Autodesk Inventor part; units mm, degrees
ref_plane "Work Plane4" through (-230, -208.6603, 455) normal (0, 0.8660254, -0.5) x (1, 0, 0)
ref_plane "Work Plane5" through (-230, -200, 450) normal (0, 0.7660444, -0.6427876) x (1, 0, 0)
ref_plane "YZ Plane" through (0, 0, 0) normal (1, 0, 0) x (0, 1, 0)
sketch "Sketch1" plane through (0, 0, 0) normal (0, 0, 1) x (1, 0, 0)
  line L0 (230, -200) -> (-230, -200)
  line L1 (-230, -200) -> (-230, 200)
  line L2 (-230, 200) -> (230, 200)
  line L3 (230, 200) -> (230, -200)
  line L4 (230, -200) -> (-230, 200) construction
  line L5 (-230, -200) -> (230, 200) construction
  line L6 (-190, 200) -> (-160.6372, 250.8579)
  line L7 (-160.6372, 250.8579) -> (139.1421, 250.8579)
  line L8 (139.1421, 250.8579) -> (190, 200)
  line L9 (139.1421, 250.8579) -> (122.8634, 211.5574) construction
  line L10 (135, 250.8579) -> (135, 240.8579) construction
  line L11 (230, 200) -> (190, 200)
  line L12 (190, 200) -> (190, 160)
  line L13 (190, 160) -> (230, 160)
  line L14 (230, 160) -> (230, 200)
  line L15 (-150, 110) -> (150, 110)
  line L16 (150, 110) -> (150, -140)
  line L17 (150, -140) -> (-150, -140)
  line L18 (-150, -140) -> (-150, 110)
  line L19 (-230, -200) -> (-190, -200)
  line L20 (-190, -200) -> (-190, -160)
  line L21 (-190, -160) -> (-230, -160)
  line L22 (-230, -160) -> (-230, -200)
  line L23 (230, -200) -> (190, -200)
  line L24 (190, -200) -> (190, -160)
  line L25 (190, -160) -> (230, -160)
  line L26 (230, -160) -> (230, -200)
  line L27 (-230, 200) -> (-190, 200)
  line L28 (-190, 200) -> (-190, 160)
  line L29 (-190, 160) -> (-230, 160)
  line L30 (-230, 160) -> (-230, 200)
  line L31 (-40, 200) -> (40, 200)
  line L32 (40, 200) -> (40, 160)
  line L33 (40, 160) -> (-40, 160)
  line L34 (-40, 160) -> (-40, 200)
  line L35 (125, 250.8579) -> (135, 250.8579)
  line L36 (135, 250.8579) -> (135, 230.8579)
  line L37 (135, 230.8579) -> (125, 230.8579)
  line L38 (125, 230.8579) -> (125, 250.8579)
  line L39 (149.1421, 240.8579) -> (142.0711, 247.9289)
  line L40 (142.0711, 247.9289) -> (127.9289, 233.7868)
  line L41 (127.9289, 233.7868) -> (134.2929, 227.4228)
  line L42 (135.7071, 227.4228) -> (149.1421, 240.8579)
  line L43 (135, 200) -> (132, 200)
  line L44 (132, 200) -> (132, 239)
  line L45 (132, 239) -> (135, 239)
  line L46 (135, 239) -> (135, 200)
  line L47 (135, 200) -> (95, 200)
  line L48 (95, 200) -> (95, 180)
  line L49 (95, 180) -> (135, 180)
  line L50 (135, 180) -> (135, 200)
  line L51 (-222, 80) -> (-132, 80)
  line L52 (-132, 80) -> (-132, -140)
  line L53 (-132, -140) -> (-222, -140)
  line L54 (-222, -140) -> (-222, 80)
  circle A0 centre (-112, -40) radius 100
  circle A1 centre (112, -40) radius 100
  line L55 (-230, -40) -> (230, -40) construction
  line L56 (-112, -40) -> (112, -40)
  arc A2 (134.2929, 227.4228) -> (135.7071, 227.4228) centre (135, 228.1299) ccw
  point P0 (0, 0)
  point P1 (0, 110)
  point P2 (0, 200)
  point P3 (135, 226.7157)
  point P4 (0, -40)
  dimension "d0" = 460
  dimension "d1" = 400
  dimension "d2" = 40
  dimension "d3" = 40
  dimension "d4" = 120
  dimension "d5" = 135
  dimension "d30" = 67.5
  dimension "d32" = 10
  dimension "d34" = 50.8579
  dimension "d35" = 40
  dimension "d36" = 40
  dimension "d37" = 300
  dimension "d38" = 250
  dimension "d39" = 60
  dimension "d40" = 40
  dimension "d41" = 40
  dimension "d42" = 40
  dimension "d43" = 40
  dimension "d44" = 40
  dimension "d45" = 40
  dimension "d46" = 80
  dimension "d47" = 40
  dimension "d48" = 10
  dimension "d50" = 10
  dimension "d51" = 3
  dimension "d52" = 39
  dimension "d53" = 40
  dimension "d54" = 20
  dimension "d55" = 55
  dimension "d56" = 105
  dimension "d57" = 90
  dimension "d58" = 220
  dimension "d59" = 8
  dimension "d60" = 20
  dimension "d61" = 55
  dimension "d63" = 200
  dimension "d64" = 160
  dimension "d65" = 118
  dimension "d66" = 1
extrude "Extrusion1" add sketch "Sketch1" along normal blind 450 contours L0 L24 L25 L3 | L0 L20 L21 L1 L29 L28 L2 L34 L33 L32 L48 L49 L50 L12 L13 L3 L25 L24 | L0 L1 L21 L20 | L13 L12 L2 L3 | L2 L46 A2 L42 L8 | L1 L2 L28 L29 | L50 L49 L48 L2 | L2 L44 L41 A2 L46 | L42 A2 L46 L36 L40 L8 | L2 L6 L7 L38 L37 L41 L44 | A2 L41 L44 L37 L46 | L40 L36 L7 L8 | L41 L37 L44 | L37 L44 L40 L45 L36 | L40 L45 L44 L41 L37 L38 L7 L36 | L36 L45 L40 | L2 L32 L33 L34 | L41 L40 L44 L37 | L40 L44 L45 | L15 L16 A1 L56 A0 L52 L51 L18 | L51 L52 A0 L18 | L18 A0 L53 L54 L51 | A1 L16 | L16 A1 | A0 L52 L18 | L18 A0 | L16 L17 A1 | A1 L17 A0 L56 | A0 L52 L17 L18 | A0 L52 | A0 L17 L52
sketch "Sketch2" plane through (0, 0, 450) normal (0, 0, 1) x (1, 0, 0)
  line L0 (-160.6372, 250.8579) -> (-190, 200)
  line L1 (-190, 200) -> (-230, 200)
  line L2 (-230, 200) -> (-230, -200)
  line L3 (-230, -200) -> (230, -200)
  line L4 (230, -200) -> (230, 200)
  line L5 (230, 200) -> (190, 200)
  line L6 (190, 200) -> (139.1421, 250.8579)
  line L7 (139.1421, 250.8579) -> (-160.6372, 250.8579)
  line L8 (230, 180) -> (-230, 180)
  point P0 (0, 0)
  dimension "d9" = 20
revolve "Revolution1" add sketch "Sketch2" angle 80 about axis through (230, 180, 450) along (1, 0, 0) contours L7 L6 L5 L4 L8 L2 L1 L0
sketch "Sketch3" plane through (-230, 180, 450) normal (0, -0.9848078, 0.1736482) x (1, 0, 0)
  line L0 (0, 20) -> (0, 0)
  line L1 (460, 0) -> (0, 0)
  line L2 (460, 0) -> (460, 20)
  line L3 (460, 20) -> (420, 20)
  line L4 (420, 20) -> (369.1421, 70.8579)
  line L5 (369.1421, 70.8579) -> (69.3628, 70.8579)
  line L6 (69.3628, 70.8579) -> (40, 20)
  line L7 (40, 20) -> (0, 20)
  point P0 (230, -474.4202)
ref_plane "Work Plane4" through (-230, -208.6603, 455) normal (0, 0.8660254, -0.5) x (1, 0, 0)
ref_plane "Work Plane3" through (-230, -200, 450) normal (0, 0.8660254, -0.5) x (1, 0, 0)
sketch "Sketch7" plane through (230, -200, 0) normal (1, 0, 0) x (0, 0, -1)
  line L0 (0, 0) -> (0, 400)
  line L1 (0, 400) -> (-450, 400)
  arc A0 (-450, 400) -> (-469.6962, 383.473) centre (-450, 380) ccw
  line L2 (-450, 380) -> (-469.6962, 383.473)
  line L3 (-450, 0) -> (-450, 380)
  line L4 (0, 0) -> (-450, 0)
  line L5 (-450, 0) -> (-537.3128, 0)
  line L6 (-537.3128, 0) -> (-469.6962, 383.473)
  arc A1 (-450, 400) -> (-469.6962, 383.473) centre (-450, 380) ccw
  line L7 (-450, 380) -> (-469.6962, 383.473)
  point P0 (0, 200)
extrude "Extrusion7" add sketch "Sketch7" against normal blind 40 contours L5 L6 L2 L3
fillet "Fillet6" radius 40 1 edges at (210, -200, 537.3128)
mirror "Mirror1" about plane through (0, 0, 0) normal (1, 0, 0) of "Extrusion7", "Fillet6"
ref_plane "Work Plane5" through (-230, -200, 450) normal (0, 0.7660444, -0.6427876) x (1, 0, 0)
sketch "Sketch9" plane through (-160.6372, 192.3043, 519.7814) normal (0, -0.9848078, 0.1736482) x (1, 0, 0)
  line L0 (-29.3628, -50.8579) -> (-29.3628, -70.8579)
  line L1 (350.6372, -70.8579) -> (-29.3628, -70.8579)
  line L2 (350.6372, -70.8579) -> (350.6372, -50.8579)
  line L3 (350.6372, -50.8579) -> (299.7793, 0)
  line L4 (299.7793, 0) -> (0, 0)
  line L5 (0, 0) -> (-29.3628, -50.8579)
  point P0 (160.6372, -545.278)
extrude "Extrusion8" add sketch "Sketch9" along normal up to surface surface through (-230, -200, 450) normal (0, 0.7660444, -0.6427876)
sketch "Sketch11" plane through (190, -200, 0) normal (-1, 0, 0) x (0, 0, 1)
  line L0 (526.0594, 63.8214) -> (508.3683, 48.9768)
  line L1 (508.3683, 48.9768) -> (450, 380)
  line L2 (450, 0) -> (450, 380)
  line L3 (450, 0) -> (489.6426, 0)
  arc A0 (489.6426, 0) -> (529.035, 46.9459) centre (489.6426, 40) ccw
  line L4 (529.035, 46.9459) -> (526.0594, 63.8214)
  line L5 (508.4341, 49.0321) -> (450, 0)
  point P0 (0, 200)
  point P1 (508.3683, 48.9768)
extrude "Extrusion9" add sketch "Sketch11" along normal up to next contours L5 L2 L1
sketch "Sketch6" plane through (-230, -200, 0) normal (-1, 0, 0) x (0, 0, 1)
  line L0 (0, 400) -> (0, 0)
  line L1 (0, 0) -> (450, 0)
  line L2 (450, 380) -> (450, 0)
  line L3 (450, 380) -> (512.6612, 24.6305)
  line L4 (531.0933, 35.2723) -> (512.6612, 24.6305)
  line L5 (469.6962, 383.473) -> (531.0933, 35.2723)
  arc A0 (469.6962, 383.473) -> (450, 400) centre (450, 380) ccw
  line L6 (0, 400) -> (450, 400)
  line L7 (512.6612, 24.6305) -> (470, 0)
  line L8 (470, 0) -> (450, 0)
  point P0 (0, 200)
equation "\"d30\" = 0.5 * d5"
properties part number "RevII Printer Envelope Study"
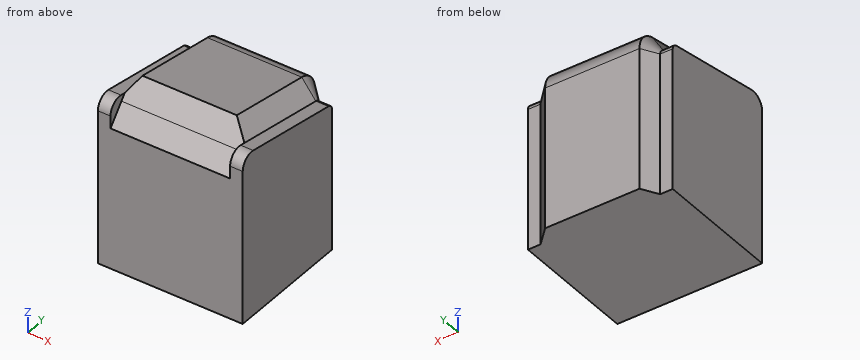
Verification items for the finished model (mm, model axes). Round coordinates to 2 decimals unless told otherwise and drop trailing zeros. Write each loop counter-clockwise with the first axis right and the second up, starting at its lowest first coordinate (ties: lowest second). Pieces come first, ordered by that corner, then holes.
(1) Material ranges on line 1 (Z direction, x = 2.5, y = 139); line 2 (Y direction, x = 209.5, z = 134); line 3 (Z direction, x = 128, y = 89.5), recorded low to high.
Returned:
line 1: z = 0 to 529.18
line 2: y = -200 to 200
line 3: z = 0 to 537.91
(2) Depth check by flat-ended pin: pin 1 Ø1.5 at (x, z) = (81, 460.5) entering from +Y; pin 2 Ø12 at (x, z) = (19, 480) entering from +Y. Enter the tip coordinate at first touch or a pass-through.
Returned:
pin 1: stops at y = 250.18
pin 2: stops at y = 246.67
(3) Section check A-A (z = 208.5). Enter the section's corners in (x, y).
Returned:
outline: (-230, -200) - (230, -200) - (230, 200) - (190, 200) - (139.14, 250.86) - (-160.64, 250.86) - (-190, 200) - (-230, 200) - close
(4) Section check C-C (x = 95). Enter the section's corners in (y, z).
Returned:
outline: (-200, 0) - (250.86, 0) - (250.86, 450) arc R70.86 ccw to (192.3, 519.78) - (-98.43, 571.05) - (-151.02, 508.37) - (-200, 450) - close
(5) Section check B-B (y = 114). Enter the section's corners in (x, z).
Returned:
outline: (-230, 0) - (230, 0) - (230, 481.95) - (190, 481.95) - (139.14, 533.59) - (-160.64, 533.59) - (-190, 481.95) - (-230, 481.95) - close
(6) Section check D-D (x = 180.5). Enter the section's corners in (y, z), plus the area to 3 significant figures.
Returned:
outline: (-200, 0) - (209.5, 0) - (209.5, 450) arc R29.5 ccw to (185.12, 479.05) - (-129.13, 534.46) - (-151.02, 508.37) - (-200, 450) - close
area: 206,000 mm2
